from build123d import *

# Parameters (mm, degrees)
BOSS_EXTRUDE2_START      = 6
BOSS_EXTRUDE2_DEPTH      = 44
CUT_EXTRUDE1_DEPTH       = 64.616841
CUT_EXTRUDE1_DEPTH_BACK  = 64.616841
SKETCH2_R                = 16.25
CUT_EXTRUDE3_DEPTH       = 64.616841
FILLET1_R                = 3
SKETCH5_W                = 35
SKETCH5_H                = 25
CUT_EXTRUDE4_DEPTH       = 10
FILLET2_R                = 3
SKETCH6_R                = 16.25
SKETCH6_R_2              = 9.5
SKETCH6_R_3              = 1.65
BOSS_EXTRUDE3_DEPTH      = 5
CUT_EXTRUDE5_DEPTH       = 68.905099
CUT_EXTRUDE5_DEPTH_BACK  = 68.905099
SKETCH7_R                = 2.25
CUT_EXTRUDE6_REACH       = 82.951
SKETCH8_R                = 1.175
BOSS_EXTRUDE4_DEPTH      = 8
BOSS_EXTRUDE4_DEPTH_BACK = 10
BOSS_EXTRUDE4_START      = -44
FILLET5_R                = 0.25
FILLET6_R                = 0.25


with BuildPart() as part:
    # Sketch1 → Boss-Extrude2 (new body)
    with BuildSketch(Plane.XY.offset(BOSS_EXTRUDE2_START)):
        with BuildLine():
            Line((-25, 0), (-25, -29.344548))
            Line((-25, -29.344548), (-25, -32.344548))
            Line((-25, -32.344548), (-20.974573, -32.344548))
            Line((-20.974573, -32.344548), (-20.974573, -35.144548))
            Line((-20.974573, -35.144548), (-15.841819, -35.144548))
            ThreePointArc((-15.841819, -35.144548), (0, -38.55), (15.841819, -35.144548))
            Line((15.841819, -35.144548), (20.974573, -35.144548))
            Line((20.974573, -35.144548), (20.974573, -32.344548))
            Line((20.974573, -32.344548), (25, -32.344548))
            Line((25, -32.344548), (25, -29.344548))
            Line((25, -29.344548), (25, 0))
            Line((25, 0), (25, 20))
            Line((25, 20), (-25, 20))
            Line((-25, 20), (-25, 0))
        make_face()
    extrude(amount=BOSS_EXTRUDE2_DEPTH)

    # Sketch2 → Cut-Extrude1 (cut, two sides: drawn at the far end of the back side and taken through both)
    with BuildSketch(Plane.XY.offset(50).offset(-CUT_EXTRUDE1_DEPTH_BACK)):
        with Locations((0, -10.3)):
            Circle(SKETCH2_R)
    extrude(amount=CUT_EXTRUDE1_DEPTH + CUT_EXTRUDE1_DEPTH_BACK, mode=Mode.SUBTRACT)

    # Sketch4 → Cut-Extrude3 (cut, through all)
    with BuildSketch(Plane.XY.offset(50)):
        with BuildLine():
            Line((-23, 18), (23, 18))
            Line((23, 18), (23, 2))
            Line((23, 2), (14.060939, 2))
            ThreePointArc((14.060939, 2), (0, 8.381542), (-14.060939, 2))
            Line((-14.060939, 2), (-23, 2))
            Line((-23, 2), (-23, 18))
        make_face()
    extrude(amount=-CUT_EXTRUDE3_DEPTH, mode=Mode.SUBTRACT)

    # Fillet1
    fillet1_edges = [part.edges().sort_by_distance(p)[0] for p in [
        (23, 18, 28),
        (23, 2, 28),
        (14.060939, 2, 28),
        (-14.060939, 2, 28),
        (-23, 2, 28),
        (-23, 18, 28),
    ]]
    fillet(fillet1_edges, radius=FILLET1_R)

    # Sketch5 → Cut-Extrude4 (cut)
    with BuildSketch(Plane(origin=(0, 20, 0), x_dir=(1, 0, 0), z_dir=(0, 1, 0))):
        with Locations((0, -37.5)):
            Rectangle(SKETCH5_W, SKETCH5_H)
    extrude(amount=-CUT_EXTRUDE4_DEPTH, mode=Mode.SUBTRACT)

    # Fillet2
    fillet2_edges = [part.edges().sort_by_distance(p)[0] for p in [
        (17.5, 19, 50),
        (17.5, 19, 25),
        (-17.5, 19, 25),
        (-17.5, 19, 50),
    ]]
    fillet(fillet2_edges, radius=FILLET2_R)

    # Sketch6 → Boss-Extrude3 (add)
    with BuildSketch(Plane.XY.offset(14)):
        with Locations((0, -10.3)):
            Circle(SKETCH6_R)
        with Locations((0, -10.3)):
            Circle(SKETCH6_R_2, mode=Mode.SUBTRACT)
        with Locations((4.446262, 1.916004)):
            Circle(SKETCH6_R_3, mode=Mode.SUBTRACT)
        with Locations((12.216004, -14.746262)):
            Circle(SKETCH6_R_3, mode=Mode.SUBTRACT)
        with Locations((-4.446262, -22.516004)):
            Circle(SKETCH6_R_3, mode=Mode.SUBTRACT)
        with Locations((-12.216004, -5.853738)):
            Circle(SKETCH6_R_3, mode=Mode.SUBTRACT)
    extrude(amount=-BOSS_EXTRUDE3_DEPTH)

    # Sketch7 → Cut-Extrude5 (cut, two sides: drawn at the far end of the back side and taken through both)
    with BuildSketch(Plane(origin=(0, 0, 0), x_dir=(0, 0, -1), z_dir=(1, 0, 0)).offset(-CUT_EXTRUDE5_DEPTH_BACK)):
        with Locations(Location((-40.3, -32, 0), (0, 0, 351.191499))):
            Circle(SKETCH7_R)
        with Locations(Location((-10.3, -32, 0), (0, 0, 351.191499))):
            Circle(SKETCH7_R)
    extrude(amount=CUT_EXTRUDE5_DEPTH + CUT_EXTRUDE5_DEPTH_BACK, mode=Mode.SUBTRACT)

    # Sketch8 → Cut-Extrude6 (cut, up to next)
    with BuildSketch(Plane(origin=(0, 20, 0), x_dir=(1, 0, 0), z_dir=(0, 1, 0)), mode=Mode.PRIVATE) as cut_extrude6_sk1:
        with Locations(Location((-4.75, -16.8, 0), (0, 0, 180))):
            Circle(SKETCH8_R)
    cut_extrude6_tool1 = extrude(cut_extrude6_sk1.sketch, amount=-CUT_EXTRUDE6_REACH, mode=Mode.PRIVATE) & part.part
    # Sketch8 → Cut-Extrude6 (cut, up to next)
    with BuildSketch(Plane(origin=(0, 20, 0), x_dir=(1, 0, 0), z_dir=(0, 1, 0)), mode=Mode.PRIVATE) as cut_extrude6_sk2:
        with Locations(Location((4.75, -16.8, 0), (0, 0, 180))):
            Circle(SKETCH8_R)
    cut_extrude6_tool2 = extrude(cut_extrude6_sk2.sketch, amount=-CUT_EXTRUDE6_REACH, mode=Mode.PRIVATE) & part.part
    add(cut_extrude6_tool1.solids().sort_by_distance((-4.75, 20, 16.8))[0], mode=Mode.SUBTRACT)
    add(cut_extrude6_tool2.solids().sort_by_distance((4.75, 20, 16.8))[0], mode=Mode.SUBTRACT)

    # Sketch9 → Boss-Extrude4 (add, two sides: drawn at the far end of the back side and taken through both)
    with BuildSketch(Plane.XY.offset(50).offset(BOSS_EXTRUDE4_START - BOSS_EXTRUDE4_DEPTH_BACK)):
        with BuildLine():
            Line((15.362267, 1), (15.362267, 10.976798))
            ThreePointArc((15.362267, 10.976798), (0, 17.081542), (-15.362267, 10.976798))
            Line((-15.362267, 10.976798), (-15.362267, 1))
            ThreePointArc((-15.362267, 1), (-13.827782, 1.306038), (-12.528102, 2.177322))
            ThreePointArc((-12.528102, 2.177322), (0, 7.381542), (12.528102, 2.177322))
            ThreePointArc((12.528102, 2.177322), (13.827782, 1.306038), (15.362267, 1))
        make_face()
        with BuildLine():
            ThreePointArc((-13.236643, 2.882992), (-13.759485, 2.464041), (-14.362267, 2.171573))
            Line((-14.362267, 2.171573), (-14.362267, 10.090161))
            ThreePointArc((-14.362267, 10.090161), (-14.272104, 10.505127), (-14.017873, 10.845264))
            ThreePointArc((-14.017873, 10.845264), (0, 16.081542), (14.017873, 10.845264))
            ThreePointArc((14.017873, 10.845264), (14.272104, 10.505127), (14.362267, 10.090161))
            Line((14.362267, 10.090161), (14.362267, 2.171573))
            ThreePointArc((14.362267, 2.171573), (13.759485, 2.464041), (13.236643, 2.882992))
            ThreePointArc((13.236643, 2.882992), (0, 8.381542), (-13.236643, 2.882992))
        make_face(mode=Mode.SUBTRACT)
    extrude(amount=BOSS_EXTRUDE4_DEPTH + BOSS_EXTRUDE4_DEPTH_BACK)

    # Fillet5
    fillet5_edges = [part.edges().sort_by_distance(p)[0] for p in [
        (0, 8.381542, -4),
        (14.272104, 10.505127, -4),
        (0, 16.081542, -4),
        (-14.272104, 10.505127, -4),
        (-13.759485, 2.464041, -4),
        (13.759485, 2.464041, -4),
        (14.362267, 6.130867, -4),
        (-14.362267, 6.130867, -4),
    ]]
    fillet(fillet5_edges, radius=FILLET5_R)

    # Fillet6
    fillet6_edges = [part.edges().sort_by_distance(p)[0] for p in [
        (-14.362267, 6.130867, 14),
        (0, 16.081542, 14),
        (14.272104, 10.505127, 14),
        (14.362267, 6.130867, 14),
        (-14.272104, 10.505127, 14),
    ]]
    fillet(fillet6_edges, radius=FILLET6_R)


solid = part.part
Build history of the part. All positions in model axes, mm. A direction names the side the tool comes from. Coordinates: 2 decimals unless noted, no trailing zeros. Order: outer loops, then holes, each group sorted by start corner. A loop starts at its lowest first (then second) coordinate and runs counter-clockwise, first axis right, second up. Notation, with made-up numbers: (56, -40) -> (79, -40) arc R13 ccw to (79, -22) -> close; hole circle Ø1 at (-2, 53.5). An arc over 180 degrees is marked (long way). One line per item, written item: value.
(1) Mould opens along Y. For faces 1 (the cylindrical face through (5.208, 0.452, 11.535)), 2 (the cylindrical face through (-13.848, 1.298, 0.93)), 3 (the flat face through (-17.5, 19, 38)) say: pulls with the +Y half, pulls with the -Y half, needs draft (parallel to the pull), parting line crosses it, or undercut.
Checked values:
face 1: undercut
face 2: pulls with the -Y half
face 3: needs draft
(2) Slice it at A-A, the plane z = 40.3. List the corners of the cut face in (x, y).
Checked values:
outline: (-25, -29.75) -> (25, -29.75) -> (25, 20) -> (17.5, 20) -> (17.5, 18) -> (20, 18) arc R3 cw to (23, 15) -> (23, 5) arc R3 cw to (20, 2) -> (15.36, 2) arc R3 cw to (13.24, 2.88) arc R18.68 ccw to (-13.24, 2.88) arc R3 cw to (-15.36, 2) -> (-20, 2) arc R3 cw to (-23, 5) -> (-23, 15) arc R3 cw to (-20, 18) -> (-17.5, 18) -> (-17.5, 20) -> (-25, 20) -> close; (-20.97, -35.14) -> (-15.84, -35.14) arc R38.55 ccw to (15.84, -35.14) -> (20.97, -35.14) -> (20.97, -34.25) -> (-20.97, -34.25) -> close; hole circle Ø32.5 at (0, -10.3)
(3) Slice it at D-D, the plane y = -31.5. List the corners of the cut face in (x, z), plus the area to 3 significant figures.
Checked values:
outline: (-25, 6) -> (25, 6) -> (25, 8.11) -> (-25, 8.11) -> close; (-25, 12.49) -> (25, 12.49) -> (25, 38.11) -> (-25, 38.11) -> close; (-25, 42.49) -> (25, 42.49) -> (25, 50) -> (-25, 50) -> close
area: 1,760 mm2
(4) Probe line 1 (Z direction, x = -19.5, y = -32); line 2 (X direction, y = -3, z = 8); line 3 (Y direction, x = 9, z = 21). List the from-to ranges inside material, lowest first. Write a range as [from, to].
Checked values:
line 1: [6, 8.05], [12.55, 38.05], [42.55, 50]
line 2: [-25, -14.52], [14.52, 25]
line 3: [-37.48, -23.83], [3.23, 6.07], [18, 20]
(5) Slice it at B-B, the plane y = -10.3. List the corners of the cut face in (x, z), plus the area to 4 significant figures.
Checked values:
outline: (-25, 6) -> (-16.25, 6) -> (-16.25, 9) -> (-9.5, 9) -> (-9.5, 14) -> (-16.25, 14) -> (-16.25, 50) -> (-25, 50) -> close; (9.5, 9) -> (16.25, 9) -> (16.25, 6) -> (25, 6) -> (25, 50) -> (16.25, 50) -> (16.25, 14) -> (9.5, 14) -> close
area: 837.5 mm2
(6) Tool access for faces 4 (the cylindrical face through (18.4, 18.96, 49.14)), 5 (the cylindrical face through (13.807, 1.315, 0.93)), 6 (the cylindrical face through (5, 19.01, 15.65)): list every direction of +Z, -Z, +X, -X, +Y, -Y with a clear straight run to the whole face (end or side of a thin tool).
Checked values:
face 4: +Z, +Y
face 5: -Z, -Y
face 6: +Y
(7) Slice it at C-C, the plane x = 0. Count the separate pieces of the cut face and the enclosed holes in it, plus the area to 3 significant figures.
Checked values:
separate pieces: 4
enclosed holes: 2
area: 737 mm2
(8) Drop flat-ended pins along their axis: pin 1 Ø12 at (x, z) = (18, 26) entering from -Y; pin 2 Ø1.4 at (y, z) = (-34, 24) entering from -X; pin 3 Ø1 at (x, z) = (-9.5, 35) entering from -Y; pin 4 Ø2.5 at (x, y) = (-4.45, -22.52) entering from -Z. Give the stop position or say it passes through.
Checked values:
pin 1: y = -36.63
pin 2: x = -20.97
pin 3: y = -37.48
pin 4: through
